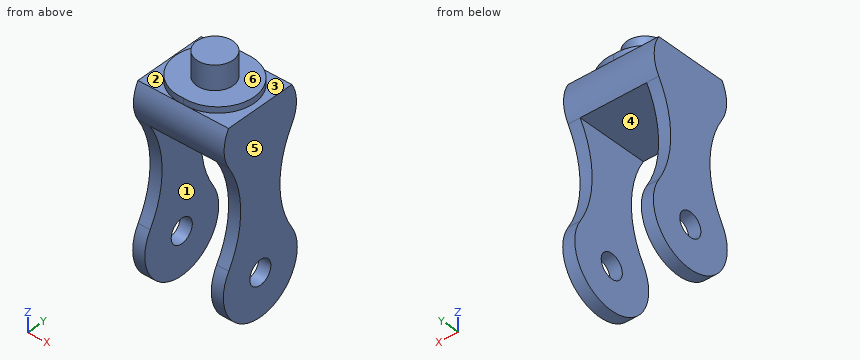
from build123d import *

# Parameters (mm, degrees)
SKETCH1_R           = 30
BOSS_EXTRUDE1_DEPTH = 5
BOSS_EXTRUDE2_DEPTH = 10
BOSS_EXTRUDE3_DEPTH = 55
SKETCH4_R           = 15
BOSS_EXTRUDE4_DEPTH = 20
SKETCH5_R           = 10
CUT_EXTRUDE1_DEPTH  = 10


with BuildPart() as part:
    # Sketch1 → Boss-Extrude1 (new body)
    with BuildSketch(Plane.XY):
        Circle(SKETCH1_R)
    extrude(amount=BOSS_EXTRUDE1_DEPTH)



with BuildPart() as body_2:
    # Sketch2 → Boss-Extrude2 (new body)
    with BuildSketch(Plane(origin=(30, 0, 0), x_dir=(0, 0, -1), z_dir=(1, 0, 0))):
        with BuildLine():
            Line((0, 30), (0, -30))
            ThreePointArc((0, -30), (15.578718077, -34.24908425), (31.103401006, -29.80663067))
            ThreePointArc((31.103401006, -29.80663067), (71.537822314, -18.507886831), (111.972243623, -29.80663067))
            ThreePointArc((111.972243623, -29.80663067), (165.159924398, 0.096684665), (111.972243623, 30))
            ThreePointArc((111.972243623, 30), (71.537822314, 18.701256161), (31.103401006, 30))
            ThreePointArc((31.103401006, 30), (15.551700503, 34.345670707), (0, 30))
        make_face()
    extrude(amount=BOSS_EXTRUDE2_DEPTH)


with BuildPart() as part_1:
    add(part.part)

    add(body_2.part)  # Boss-Extrude3 merges body 2
    # Sketch3 → Boss-Extrude3 (add)
    with BuildSketch(Plane.ZY.offset(-30)):
        with BuildLine():
            Line((-31.103401006, 30), (-31.103401006, -29.80663067))
            ThreePointArc((-31.103401006, -29.80663067), (-15.578718077, -34.24908425), (0, -30))
            Line((0, -30), (0, 30))
            ThreePointArc((0, 30), (-15.551700503, 34.345670707), (-31.103401006, 30))
        make_face()
    extrude(amount=BOSS_EXTRUDE3_DEPTH)

    # Mirror1: part across plane


with BuildPart() as part_2:
    add(part_1.part)
    add(part_1.part.mirror(Plane.ZY.offset(-2.5)))

    # Sketch4 → Boss-Extrude4 (add)
    with BuildSketch(Plane.XY.offset(5)):
        with Locations((2.5, 0)):
            Circle(SKETCH4_R)
    extrude(amount=BOSS_EXTRUDE4_DEPTH)

    # Sketch5 → Cut-Extrude1 (cut)
    with BuildSketch(Plane.ZY.offset(-30)):
        with Locations((-130.159924398, 0.096684665)):
            Circle(SKETCH5_R)
    cut_extrude1 = extrude(amount=-CUT_EXTRUDE1_DEPTH, mode=Mode.SUBTRACT)

    # Mirror2: Cut-Extrude1 across plane
    add(cut_extrude1.mirror(Plane.ZY.offset(-2.5)), mode=Mode.SUBTRACT)


solid = part_2.part
Input: part model. Units: mm. Frame: model coordinates. Face numbers are marked on the shaded views. A direction names the side the tool comes from. Give positions to 0.01 mm unless a question says otherwise; leave off trailing zeros. Loops run counter-clockwise (first coordinate to the right, second up) from the corner with the lowest first, then second, coordinate; pieces in that order, holes last. Notation, with made-up numbers: (-3, 25) -> (3, 25) arc R8 cw to (3, 40) -> close; hole circle Ø6 at (22, -3). An arc over 180 degrees is marked (long way). Answer as a JSON object with one key per item and string values. Group by question number.
Item 1: Cut plane C-C, the plane x = -5.5. Return the cut outline in (y, z).
Item 2: Pin query (flat end, axial travel): P1, Ø12, axis at x = -20, y = 0, coming from the +Z side; P2, Ø18, axis at y = 0.1, z = -130.16, coming from the +X side; P3, Ø12, axis at x = -11, z = -19, coming from the +Y side; P4, Ø8, axis at x = 16, y = 0, coming from the -Z side. Return the tip coordinate at first contact, or that it passes through.
Item 3: Reachability of the marked faces 1, 2 and 3 from +Z, -Z, +X, -X, +Y, -Y: full face, straight path, thin tool, end or side. Return the list, or none.
Item 4: Cut plane B-B, the plane y = 7.5. Return the cut outline in (x, z).
Item 5: Line query: probe 1 along X at (y, z) = (10, -42); probe 2 along Z at (x, y) = (-2.5, 13); probe 3 along Z at (x, y) = (23, -5.5). Output: solid intervals per line, ascending.
Item 6: Cut plane D-D, the plane y = -7.5. Return the cut outline in (x, z).
Item 7: Pull-direction query (X, two-part tool) for the marked faces 4, 5 and 6; classes: released by +X, released by -X, zero draft, split by the parting line, or undercut.
Item 8: Cut plane A-A, the plane z = -71.5. Return the cut outline in (x, y).
Checks:
{
 "1": {"outline": "(-30, 0) arc R30 ccw to (-29.81, -31.1) -> (30, -31.1) arc R30 ccw to (30, 0) -> (29.49, 0) -> (29.49, 5) -> (12.69, 5) -> (12.69, 25) -> (-12.69, 25) -> (-12.69, 5) -> (-29.49, 5) -> (-29.49, 0) -> close"},
 "2": {"P1": "stops at z = 5", "P2": "passes through", "P3": "stops at y = 34.35", "P4": "stops at z = -31.1"},
 "3": {"face 1": "-Z, +Y, -Y", "face 2": "+Z, -X", "face 3": "+Z, +X"},
 "4": {"outline": "(-35, -164.37) -> (-25, -164.37) -> (-25, -136.88) -> (-35, -136.88) -> close; (-35, -123.44) -> (-25, -123.44) -> (-25, -31.1) -> (30, -31.1) -> (30, -123.44) -> (40, -123.44) -> (40, 0) -> (34.05, 0) -> (34.05, 5) -> (15.49, 5) -> (15.49, 25) -> (-10.49, 25) -> (-10.49, 5) -> (-29.05, 5) -> (-29.05, 0) -> (-35, 0) -> close; (30, -164.37) -> (40, -164.37) -> (40, -136.88) -> (30, -136.88) -> close"},
 "5": {"probe 1": "x = -35 to -25, 30 to 40", "probe 2": "z = -31.1 to 25", "probe 3": "z = -31.1 to 5"},
 "6": {"outline": "(-35, -164.33) -> (-25, -164.33) -> (-25, -136.66) -> (-35, -136.66) -> close; (-35, -123.66) -> (-25, -123.66) -> (-25, -31.1) -> (30, -31.1) -> (30, -123.66) -> (40, -123.66) -> (40, 0) -> (34.05, 0) -> (34.05, 5) -> (15.49, 5) -> (15.49, 25) -> (-10.49, 25) -> (-10.49, 5) -> (-29.05, 5) -> (-29.05, 0) -> (-35, 0) -> close; (30, -164.33) -> (40, -164.33) -> (40, -136.66) -> (30, -136.66) -> close"},
 "7": {"face 4": "undercut", "face 5": "released by +X", "face 6": "zero draft"},
 "8": {"outline": "(-35, -18.51) -> (-25, -18.51) -> (-25, 18.7) -> (-35, 18.7) -> close; (30, -18.51) -> (40, -18.51) -> (40, 18.7) -> (30, 18.7) -> close"}
}
